Check sheet for the drawn part. Datum: minimum x, y, z corner. Units: mm. A direction names the side the tool comes from. Round coordinates to 2 decimals unless told otherwise and drop trailing zeros. Write each loop counter-clockwise with the first axis right and the second up, starting at its lowest first coordinate (ties: lowest second). Pieces come first, ordered by that corner, then holes. Notation, with made-up numbers: (-9, 7.5) -> (12, 7.5) arc R20 ccw to (12, 12.5) -> close; hole circle Ø1 at (21.25, -36.75). An arc over 180 degrees is marked (long way). Use CSV: the item, a comma, the result in double quotes.
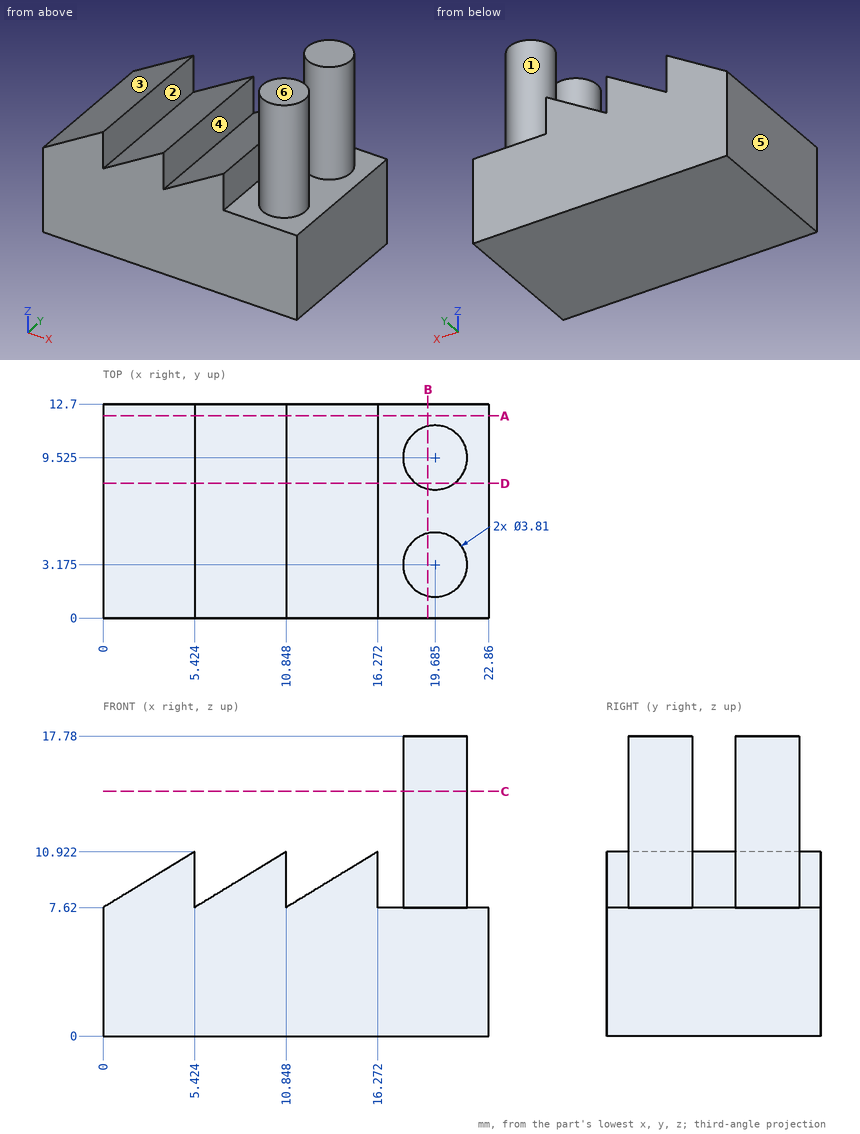
Q1. Section check A-A (y = 12). Record the cut outline in (x, z).
Filled in:
outline,"(0, 0) -> (22.86, 0) -> (22.86, 7.62) -> (16.27, 7.62) -> (16.27, 10.92) -> (10.85, 7.62) -> (10.85, 10.92) -> (5.42, 7.62) -> (5.42, 10.92) -> (0, 7.62) -> close"
Q2. Access from +Z, -Z, +X, -X, +Y, -Y to the whole of each face (thin tool, end or side, straight path). Record for the marked faces 1, 2 and 3.
Filled in:
face 1,"+Z"
face 2,"+Z, +Y, -Y"
face 3,"+Z, -X, +Y, -Y"
Q3. Material ranges on L1, parallel to X at y = 12.25, z = 8 (1 decimal); L2, parallel to X at y = 3.25, z = 10 (1 decimal); L3, parallel to Y at x = 20.25, z = 11.5, recorded low to high.
Filled in:
L1,"0.6 to 5.4, 6 to 10.8, 11.5 to 16.3"
L2,"3.9 to 5.4, 9.3 to 10.8, 14.8 to 16.3, 17.8 to 21.6"
L3,"1.36 to 4.99, 7.71 to 11.34"
Q4. Section check B-B (x = 19.25). Record the cut outline in (y, z), plus the area to 3 significant figures.
Filled in:
outline,"(0, 0) -> (12.7, 0) -> (12.7, 7.62) -> (11.38, 7.62) -> (11.38, 17.78) -> (7.67, 17.78) -> (7.67, 7.62) -> (5.03, 7.62) -> (5.03, 17.78) -> (1.32, 17.78) -> (1.32, 7.62) -> (0, 7.62) -> close"
area,"172 mm²"
Q5. Section check C-C (z = 14.5). Record the cut outline in (x, y) (3 decimals).
Filled in:
outline,"circle Ø3.81 at (19.685, 3.175); circle Ø3.81 at (19.685, 9.525)"
Q6. Section check D-D (y = 8). Record the cut outline in (x, z).
Filled in:
outline,"(0, 0) -> (22.86, 0) -> (22.86, 7.62) -> (20.83, 7.62) -> (20.83, 17.78) -> (18.54, 17.78) -> (18.54, 7.62) -> (16.27, 7.62) -> (16.27, 10.92) -> (10.85, 7.62) -> (10.85, 10.92) -> (5.42, 7.62) -> (5.42, 10.92) -> (0, 7.62) -> close"
Q7. Mould release check, pull along X, two halves, no side actions. Record for the marked faces 4, 5 and 6: released by +X, released by -X, zero draft, split by the parting line, or undercut.
Filled in:
face 4,"undercut"
face 5,"released by -X"
face 6,"zero draft"
Q8. Go/stop test with flat-tipped pins: P1, Ø4, axis at y = 6, z = 12.5, coming from the -X side; P2, Ø1.5, axis at x = 8, y = 1.5, coming from the +Z side (1 decimal); P3, Ø1.7, axis at y = 3.5, z = 9, coming from the +X side. Record where each tip stops, or that it passes through.
Filled in:
P1,"x = 4.73"
P2,"z = 9.6"
P3,"x = 21.59"
